from build123d import *

# Parameters (mm, degrees)
BOSS_EXTRUDE1_DEPTH = 19.4


with BuildPart() as part:
    # Sketch1 → Boss-Extrude1 (new body)
    with BuildSketch(Plane.XY):
        Polygon((0, 19.629909152), (-17, 9.814954576), (-17, -9.814954576), (0, -19.629909152), (17, -9.814954576), (17, 9.814954576), align=None)
    extrude(amount=-BOSS_EXTRUDE1_DEPTH)

    # Sketch4 → Cut-Revolve1 (revolve, cut)
    with BuildSketch(Plane(origin=(0, 0, 0), x_dir=(0, 0, -1), z_dir=(1, 0, 0))):
        Polygon((19.4, 19.629909152), (17.131065893, 19.629909152), (19.4, 15.7), align=None)
        Polygon((0, 19.629909152), (2.268934107, 19.629909152), (0, 15.7), align=None)
    revolve(axis=Axis((0, 0, 0), (0, 0, -1)), mode=Mode.SUBTRACT)

    # Sketch5 → Cut-Revolve2 (revolve, cut)
    with BuildSketch(Plane(origin=(0, 0, 0), x_dir=(0, 0, -1), z_dir=(1, 0, 0))):
        Polygon((0, 0), (0, 11.25), (1.5, 9.75), (17.9, 9.75), (19.4, 11.25), (19.4, 0), align=None)
    revolve(axis=Axis((0, 0, 0), (0, 0, -1)), mode=Mode.SUBTRACT)


solid = part.part
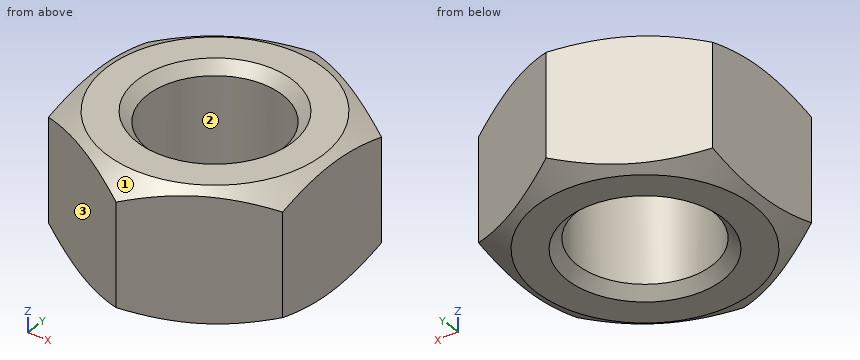
Could you check a few things on this model? Use its own coordinates, in mm. Face numbers are marked on the shaded views. Coordinates: 2 decimals unless noted, no trailing zeros. Write each loop counter-clockwise with the first axis right and the second up, starting at its lowest first coordinate (ties: lowest second). Pieces come first, ordered by that corner, then holes. Notation, with made-up numbers: M 9.25,49 L 17.25,49 A19 cw 17.25,77 Z; hole C 88.5,42 d7. An arc over 180 degrees is marked long. One line per question, with ' | ' between items.
1) If we mould it in two halves opening along X, with no side actions, what happens to the marked faces 1, 2 and 3? For each: released by +X, released by -X, zero draft, split by the parting line, or undercut.
Checks:
face 1: split by the parting line | face 2: undercut | face 3: released by -X
2) I need wall thicknesses on probe 1 along X at (y, z) = (0, -7.5); probe 2 along Y at (x, z) = (-3, -12.25); probe 3 along X at (y, z) = (-5, -14.5). Which ranges of each line are inside material? Lowest first, please. Write a range as [from, to].
Checks:
probe 1: [-17, -9.75], [9.75, 17] | probe 2: [-17.9, -9.28], [9.28, 17.9] | probe 3: [-17, -8.37], [8.37, 17]
3) For pin 1 Ø12 at (x, y) = (0, 9.5) entering from +Z; pin 2 Ø5 at (x, z) = (3, -16) entering from +Y; pin 3 Ø5 at (x, z) = (4, -6) entering from +Y, each with a flat end and sliding along its axis, tell me the tip position at first contact or that it passes through.
Checks:
pin 1: z = 0 | pin 2: y = 19.34 | pin 3: y = 18.76
4) Imagine slicing it at A-A, the plane y = 0. Write out the boundary of the cut face in (x, z), and give its area (3 significant figures).
Checks:
outline: M -17,-18.65 L -15.7,-19.4 L -11.25,-19.4 L -9.75,-17.9 L -9.75,-1.5 L -11.25,0 L -15.7,0 L -17,-0.75 Z; M 9.75,-17.9 L 11.25,-19.4 L 15.7,-19.4 L 17,-18.65 L 17,-0.75 L 15.7,0 L 11.25,0 L 9.75,-1.5 Z | area: 275 mm²
5) Imagine slicing it at B-B, the plane z = -15.5. Write out the boundary of the cut face in (x, y), and give its area (3 significant figures).
Checks:
outline: M -17,-9.81 L 0,-19.63 L 17,-9.81 L 17,9.81 L 0,19.63 L -17,9.81 Z; hole C 0,0 d19.5 | area: 702 mm²
